from build123d import *

# Parameters (mm, degrees)
SKETCH_1_W          = 57.12
SKETCH_1_H          = 30
EXTRUDE_1_DEPTH     = 15
SKETCH_2_R          = 1.75
CUT_EXTRUDE_1_DEPTH = 61.93188328
SKETCH_4_R          = 18.5
EXTRUDE_4_DEPTH     = 15
SKETCH_5_R          = 18.5
SKETCH_5_R_2        = 12.5
EXTRUDE_5_DEPTH     = 7
SKETCH_6_R          = 18.5
SKETCH_6_R_2        = 17.5
EXTRUDE_6_DEPTH     = 1
FILLET_1_R          = 3
SKETCH_7_R          = 2
CUT_EXTRUDE_2_DEPTH = 71.387692106
CUT_EXTRUDE_3_DEPTH = 71.387692168
FILLET_2_R          = 10
SKETCH_9_W          = 41.12
SKETCH_9_H          = 10
CUT_EXTRUDE_4_DEPTH = 66.931203604
FILLET_3_R          = 5


with BuildPart() as part:
    # ｽｹｯﾁ1 → ﾎﾞｽ - 押し出し1 (new body)
    with BuildSketch(Plane.XY):
        Rectangle(SKETCH_1_W, SKETCH_1_H)
    extrude(amount=EXTRUDE_1_DEPTH)

    # ｽｹｯﾁ2 → ｶｯﾄ - 押し出し1 (cut, through all)
    with BuildSketch(Plane.ZY.offset(28.56)):
        with Locations((7.5, 10)):
            Circle(SKETCH_2_R)
        with Locations(Location((7.5, -10, 0), (0, 0, 180))):
            Circle(SKETCH_2_R)
    extrude(amount=-CUT_EXTRUDE_1_DEPTH, mode=Mode.SUBTRACT)

    # ｽｹｯﾁ4 → ﾎﾞｽ - 押し出し4 (add, through all)
    with BuildSketch(Plane.XY.offset(15)):
        with BuildLine():
            Line((-28.56, 34), (-28.56, 15))
            Line((-28.56, 15), (28.56, 15))
            Line((28.56, 15), (28.56, 34))
            ThreePointArc((28.56, 34), (0, 62.56), (-28.56, 34))
        make_face()
        with Locations((0, 34)):
            Circle(SKETCH_4_R, mode=Mode.SUBTRACT)
    extrude(amount=-EXTRUDE_4_DEPTH)

    # ｽｹｯﾁ5 → ﾎﾞｽ - 押し出し5 (add)
    with BuildSketch(Plane.XY.offset(15)):
        with Locations((0, 34)):
            Circle(SKETCH_5_R)
        with Locations((0, 34)):
            Circle(SKETCH_5_R_2, mode=Mode.SUBTRACT)
    extrude(amount=-EXTRUDE_5_DEPTH)

    # ｽｹｯﾁ6 → ﾎﾞｽ - 押し出し6 (add)
    with BuildSketch(Plane(origin=(0, 0, 8), x_dir=(-1, 0, 0), z_dir=(0, 0, -1))):
        with Locations(Location((0, 34, 0), (0, 0, 180))):
            Circle(SKETCH_6_R)
        with Locations((0, 34)):
            Circle(SKETCH_6_R_2, mode=Mode.SUBTRACT)
    extrude(amount=EXTRUDE_6_DEPTH)

    # ﾌｨﾚｯﾄ1
    fillet_1_edges = [part.edges().sort_by_distance(p)[0] for p in [
        (28.56, -15, 7.5),
        (-28.56, -15, 7.5),
    ]]
    fillet(fillet_1_edges, radius=FILLET_1_R)

    # ｽｹｯﾁ7 → ｶｯﾄ - 押し出し2 (cut, through all)
    with BuildSketch(Plane(origin=(0, 0, 0), x_dir=(-1, 0, 0), z_dir=(0, 0, -1))):
        with Locations((0, 9.5)):
            Circle(SKETCH_7_R)
        with Locations((-21.217622393, 21.75)):
            Circle(SKETCH_7_R)
        with Locations(Location((21.217622393, 21.75, 0), (0, 0, 180))):
            Circle(SKETCH_7_R)
    extrude(amount=-CUT_EXTRUDE_2_DEPTH, mode=Mode.SUBTRACT)

    # ｽｹｯﾁ8 → ｶｯﾄ - 押し出し3 (cut, through all)
    with BuildSketch(Plane(origin=(0, 0, 0), x_dir=(-1, 0, 0), z_dir=(0, 0, -1))):
        with BuildLine():
            Line((-28.56, 34), (-28.56, 21.75))
            Line((-28.56, 21.75), (-23.5, 34))
            ThreePointArc((-23.5, 34), (0, 57.5), (23.5, 34))
            Line((23.5, 34), (28.56, 21.75))
            Line((28.56, 21.75), (28.56, 34))
            ThreePointArc((28.56, 34), (0, 62.56), (-28.56, 34))
        make_face()
    extrude(amount=-CUT_EXTRUDE_3_DEPTH, mode=Mode.SUBTRACT)

    # ﾌｨﾚｯﾄ2
    fillet_2_edges = [part.edges().sort_by_distance(p)[0] for p in [
        (23.5, 34, 7.5),
        (28.56, 21.75, 7.5),
        (-28.56, 21.75, 7.5),
        (-23.5, 34, 7.5),
    ]]
    fillet(fillet_2_edges, radius=FILLET_2_R)

    # ｽｹｯﾁ9 → ｶｯﾄ - 押し出し4 (cut, through all)
    with BuildSketch(Plane(origin=(0, 0, 0), x_dir=(-1, 0, 0), z_dir=(0, 0, -1))):
        Rectangle(SKETCH_9_W, SKETCH_9_H)
    extrude(amount=-CUT_EXTRUDE_4_DEPTH, mode=Mode.SUBTRACT)

    # ﾌｨﾚｯﾄ3
    fillet_3_edges = [part.edges().sort_by_distance(p)[0] for p in [
        (-20.56, 5, 7.5),
        (-20.56, -5, 7.5),
        (20.56, 5, 7.5),
        (20.56, -5, 7.5),
    ]]
    fillet(fillet_3_edges, radius=FILLET_3_R - 0.0001)  # a hair under: the kernel refuses the full size


solid = part.part
Design review of the part built by this model. Coordinates are the model's own, in mm. A direction names the side the tool comes from. Round coordinates to 2 decimals unless told otherwise and drop trailing zeros. Loops run counter-clockwise (first coordinate to the right, second up) from the corner with the lowest first, then second, coordinate; pieces in that order, holes last. Notation, with made-up numbers: M 81,78.25 L 126,78.25 A28 cw 126,117.25 Z; hole C 9,42.25 d3. An arc over 180 degrees is marked long. Answer as a JSON object with one key per item and string values.
Item 1: The part is to be moulded in two halves that separate along Y. For faces 1 (the cylindrical face through (27.7, -14.1, 7.6)), 2 (the cylindrical face through (-14.68, 22.74, 3.55)), 3 (the flat face through (0, 14, 0)), say which applies: pulls with the +Y half, pulls with the -Y half, needs draft (parallel to the pull), parting line crosses it, or undercut.
Answer sheet:
{"face 1": "pulls with the -Y half", "face 2": "undercut", "face 3": "needs draft"}
Item 2: We need section A-A on y = -10. Give the boundary of the cut face in (x, z).
Answer sheet:
{"outline": "M -28.56,0 L 28.56,0 L 28.56,5.75 L -28.56,5.75 Z; M -28.56,9.25 L 28.56,9.25 L 28.56,15 L -28.56,15 Z"}
Item 3: Clearance check with flat-ended pins moving along their axes: P1, Ø4, axis at y = 29.5, z = 7.5, coming from the -X side; P2, Ø2, axis at y = 29, z = 12, coming from the -X side; P3, Ø2, axis at y = 43, z = 13.5, coming from the -X side. State where each tip first meets the part, or that it passes through.
Answer sheet:
{"P1": "stops at x = -26.18", "P2": "stops at x = -25.98", "P3": "stops at x = -22.1"}
Item 4: Wall thickness on L1, parallel to Y at x = 0, z = 7.5; L2, parallel to Y at x = 0, z = 11; L3, parallel to Y at x = 17, z = 6.5: over which ranges is each line inside the solid? List them lowest first. Write a range as from..to.
Answer sheet:
{"L1": "y = -15..-11.75, -8.25..-5, 5..7.5, 11.75..16.5, 51.5..57.5", "L2": "y = -15..-5, 5..7.5, 11.5..21.5, 46.5..57.5", "L3": "y = -15..-11.44, -8.56..-4.79, 4.79..8.56, 11.44..26.7, 41.3..50.22"}
Item 5: We need section D-D on x = 8. Give the boundary of the cut face in (y, z), and give its area (3 significant figures).
Answer sheet:
{"outline": "M -15,0 L -5,0 L -5,15 L -15,15 Z; M 5,0 L 17.32,0 L 17.32,7 L 18.44,7 L 18.44,8 L 24.4,8 L 24.4,15 L 5,15 Z; M 43.6,8 L 49.56,8 L 49.56,7 L 50.68,7 L 50.68,0 L 56.1,0 L 56.1,15 L 43.6,15 Z; hole C -10,7.5 d3.5; hole C 10,7.5 d3.5", "area": "498 mm^2"}
Item 6: We need section B-B on x = 0. Give the boundary of the cut face in (y, z).
Answer sheet:
{"outline": "M -15,0 L -5,0 L -5,15 L -15,15 Z; M 5,0 L 7.5,0 L 7.5,15 L 5,15 Z; M 11.5,0 L 15.5,0 L 15.5,7 L 16.5,7 L 16.5,8 L 21.5,8 L 21.5,15 L 11.5,15 L 11.5,8.4 A1.75 cw 11.5,6.6 Z; M 46.5,8 L 51.5,8 L 51.5,7 L 52.5,7 L 52.5,0 L 57.5,0 L 57.5,15 L 46.5,15 Z; hole C -10,7.5 d3.5"}
Item 7: We need section C-C on z = 10.25. State how many separate pieces and enclosed holes the cut face has, and give its area (3 significant figures).
Answer sheet:
{"separate pieces": "1", "enclosed holes": "5", "area": "2,680 mm^2"}
Item 8: Machinability: for faces 4 (the cylindrical face through (-19.13, -3.5, 7.6)), 5 (the cylindrical face through (-23.695, 33.869, 7.605)), 6 (the flat face through (11, 26, 8)), which of the approach directions +Z, -Z, +X, -X, +Y, -Y give a long, thin tool a straight path to every point of the face, cutting with its end or side? Answer none if there is none.
Answer sheet:
{"face 4": "+Z, -Z", "face 5": "+Z, -Z, -X, +Y", "face 6": "-Z"}
